Part model, mm, in its own coordinate system. A direction names the side the tool comes from. Round coordinates to 2 decimals unless told otherwise and drop trailing zeros. Loops run counter-clockwise (first coordinate to the right, second up) from the corner with the lowest first, then second, coordinate; pieces in that order, holes last. Notation, with made-up numbers: M 61,34.5 L 96,34.5 A12 ccw 96,38.5 Z; hole C 29.5,6 d7. An arc over 180 degrees is marked long. Answer as CSV lines item,"result". Start each with the question number.
Item 1: Drop flat-ended pins along their axis: pin 1 Ø3 at (y, z) = (65.5, 14.5) entering from +X; pin 2 Ø5 at (y, z) = (140, 4.5) entering from -X; pin 3 Ø10 at (y, z) = (229, 16) entering from -X. Give the stop position or say it passes through.
Item 2: Band-saw the part on C-C (y = 175.5). Give the cut face in (x, z), and give its area (3 significant figures).
Item 3: Which spindle directions (+Z, -Z, +X, -X, +Y, -Y) get a long thin tool onto all of the face, cutting with end or side? Do faces 4 (the cylindrical face through (-5080.96, 314.8, 9.39)), 5 (the flat face through (-5222, 0, 9)). Say none if no direction does.
Item 4: Mould opens along Y. For faces 1 (the flat face through (-5007, 203.073, 10)), 2 (the flat face through (-4972.245, 100.115, 9.658)), 3 (the flat face through (-5222, 533.146, 9)) say: pulls with the +Y half, pulls with the -Y half, needs draft (parallel to the pull), parting line crosses it, or undercut.
Item 5: Band-saw the part on A-A (x = -5032). Give the cut face in (y, z).
Item 6: Wall check: line 1 (Y direction, x = -5013.5, z = 14); line 2 (X direction, y = 489.5, z = 14); line 3 (X direction, y = 46, z = 2.5). Give the ranges that are in metal, low to high.
Item 7: Band-saw the part on B-B (z = 12.5). Give the cut face in (x, y), and give its area (3 significant figures).
```python
from build123d import *

# Parameters (mm, degrees)
SKETCH1_W           = 493.106084352
SKETCH1_H           = 533.146
BOSS_EXTRUDE1_DEPTH = 19.05
BOSS_EXTRUDE3_DEPTH = 533.146
CUT_EXTRUDE1_DEPTH  = 5496.210802379
SKETCH5_W           = 127
SKETCH5_H           = 127
CUT_EXTRUDE2_DEPTH  = 5496.210802379
FILLET1_R           = 50.8


with BuildPart() as part:
    # Sketch1 → Boss-Extrude1 (new body)
    with BuildSketch(Plane.XY):
        with Locations((-5222.700490325, 266.573)):
            Rectangle(SKETCH1_W, SKETCH1_H)
    extrude(amount=BOSS_EXTRUDE1_DEPTH)

    # Boss-Extrude3: read off the stored shape, not the designer's step
    # Boss-Extrude3 outline → Boss-Extrude3 (add)
    with BuildSketch(Plane(origin=(0, 0, 0), x_dir=(1, 0, 0), z_dir=(0, 1, 0))):
        Polygon((-4976.147448149, -19.05), (-4968.450748546, -19.05), (-4976.147448148, 0), align=None)
    extrude(amount=BOSS_EXTRUDE3_DEPTH)

    # Sketch2 → Cut-Extrude1 (cut, through all)
    with BuildSketch(Plane(origin=(0, 533.146, 0), x_dir=(1, 0, 0), z_dir=(0, 1, 0))):
        Polygon((-5469.253532501, 0), (-5461.556832899, -19.05), (-5469.253532501, -19.05), align=None)
    extrude(amount=-CUT_EXTRUDE1_DEPTH, mode=Mode.SUBTRACT)

    # Sketch5 → Cut-Extrude2 (cut, through all)
    with BuildSketch(Plane.XY.offset(19.05)):
        with Locations((-5031.950748546, 266.573)):
            Rectangle(SKETCH5_W, SKETCH5_H)
    extrude(amount=-CUT_EXTRUDE2_DEPTH, mode=Mode.SUBTRACT)

    # Fillet1
    fillet1_edges = [part.edges().sort_by_distance(p)[0] for p in [
        (-5095.450748546, 330.073, 9.525),
        (-5095.450748546, 203.073, 9.525),
    ]]
    fillet(fillet1_edges, radius=FILLET1_R)


solid = part.part
```
Answer block:
1,pin 1,"stops at x = -4969.68"
1,pin 2,"stops at x = -5468.45"
1,pin 3,"stops at x = -5464.81"
2,outline,"M -5469.25,0 L -4976.15,0 L -4968.45,19.05 L -5461.56,19.05 Z"
2,area,"9,390 mm^2"
3,face 4,"+Z, -Z, +X"
3,face 5,"+Z, -Z, +X, -X, -Y"
4,face 1,"undercut"
4,face 2,"needs draft"
4,face 3,"pulls with the +Y half"
5,outline,"M 0,0 L 203.07,0 L 203.07,19.05 L 0,19.05 Z; M 330.07,0 L 533.15,0 L 533.15,19.05 L 330.07,19.05 Z"
6,line 1,"y = 0 to 203.07, 330.07 to 533.15"
6,line 2,"x = -5463.6 to -4970.49"
6,line 3,"x = -5468.24 to -4975.14"
7,outline,"M -5464.2,0 L -4971.1,0 L -4971.1,203.07 L -5044.65,203.07 A50.8 cw -5095.45,253.87 L -5095.45,279.27 A50.8 cw -5044.65,330.07 L -4971.1,330.07 L -4971.1,533.15 L -5464.2,533.15 Z"
7,area,"248,000 mm^2"
